```python
from build123d import *

# Parameters (mm, degrees)
EXTRUDE1_DEPTH = 3.81
FILLET1_R      = 0.381
CHAMFER1_SIZE  = 0.79502


with BuildPart() as part:
    # Sketch1 → Revolve1 (revolve)
    with BuildSketch(Plane.XY):
        Polygon((25.4, 0), (25.4, 3.1115), (-19.05, 3.1115), (-19.05, 4.699), (-25.4, 4.699), (-25.4, 0), align=None)
    revolve(axis=Axis((-24.504761338, 0, 0), (1, 0, 0)))

    # Sketch2 → Extrude1 (cut)
    with BuildSketch(Plane.ZY.offset(25.4)):
        Polygon((0, 2.749630657), (-2.38125, 1.374815329), (-2.38125, -1.374815329), (0, -2.749630657), (2.38125, -1.374815329), (2.38125, 1.374815329), align=None)
    extrude(amount=-EXTRUDE1_DEPTH, mode=Mode.SUBTRACT)

    # Fillet1
    fillet1_edges = [part.edges().sort_by_distance(p)[0] for p in [
        (-25.4, -4.699, 0),
        (-19.05, -4.699, 0),
    ]]
    fillet(fillet1_edges, radius=FILLET1_R)

    # Chamfer1
    chamfer1_edges = [part.edges().sort_by_distance(p)[0] for p in [
        (25.4, -3.1115, 0),
    ]]
    chamfer(chamfer1_edges, length=CHAMFER1_SIZE)


solid = part.part
```
Source: CAD feature listing. Evaluate the final solid. Frame: model axes, mm. A direction names the side the tool comes from. Round coordinates to 2 decimals unless told otherwise and drop trailing zeros. Loops run counter-clockwise (first coordinate to the right, second up) from the corner with the lowest first, then second, coordinate; pieces in that order, holes last. Notation, with made-up numbers: M 3,5.25 L 56,5.25 A23 ccw 56,39.25 Z; hole C 8,-36.5 d1. An arc over 180 degrees is marked long. Use a Markdown table: item, result. Add a question column.
1. Cut plane A-A, the plane y = 0. Output: boundary loops of the cut face in (x, z).
2. Pull-direction query (Y, two-part tool) for faces 4 (the flat face through (-23.522, -2.072, 1.174)), 5 (the flat face through (25.4, 0, 0)), 6 (the cylindrical face through (2.47, -0.67, -3.04)); classes: +Y half, -Y half, draft (parallel to the pull), parting line (faces both ways), or undercut.
3. Set-up query: faces 1 (the cylindrical face through (-22.26, -0.61, 4.66)), 2 (the flat face through (-19.05, -3, -2)), 3 (the flat face through (-21.59, 0, 0)). Return all of +Z, -Z, +X, -X, +Y, -Y with unobstructed straight access to the full face (end or side cutting, diameter ignored); none if empty.
4. Ray query, line 1 along X through (y, z) = (3.75, 1); line 2 along Z through (x, y) = (-6, 2). Return the intervals inside material, ascending. Write a range as [from, to].
5. Contact query for flat-ended pins moving along their axis: pin 1 (1 mm diameter, centred on x = 3, y = -2, fed in from -Z); pin 2 (1 mm diameter, centred on x = 2.5, z = 3, fed in from +Y); pin 3 (1 mm diameter, centred on x = -4, z = 2.5, fed in from +Y). Output: stop coordinate, or through.
6. Cut plane B-B, the plane x = -18.5. Output: boundary loops of the cut face in (y, z), and give its area (3 significant figures).
Solution:
| question | item | result |
|---|---|---|
| 1 | outline | M -25.4,-4.32 A0.38 ccw -25.02,-4.7 L -19.43,-4.7 A0.38 ccw -19.05,-4.32 L -19.05,-3.11 L 24.6,-3.11 L 25.4,-2.32 L 25.4,2.32 L 24.6,3.11 L -19.05,3.11 L -19.05,4.32 A0.38 ccw -19.43,4.7 L -25.02,4.7 A0.38 ccw -25.4,4.32 L -25.4,2.38 L -21.59,2.38 L -21.59,-2.38 L -25.4,-2.38 Z |
| 2 | face 4 | undercut |
| 2 | face 5 | draft |
| 2 | face 6 | parting line |
| 3 | face 1 | +X, -X |
| 3 | face 2 | +X |
| 3 | face 3 | -X |
| 4 | line 1 | x = [-25.4, -19.05] |
| 4 | line 2 | z = [-2.38, 2.38] |
| 5 | pin 1 | stops at z = -2.73 |
| 5 | pin 2 | stops at y = 1.85 |
| 5 | pin 3 | stops at y = 2.38 |
| 6 | outline | C 0,0 d6.22 |
| 6 | area | 30.4 mm2 |
